```python
from build123d import *

# Parameters (mm, degrees)
SKETCH_1_R      = 4.25
EXTRUDE_1_DEPTH = 2.8
FILLET_1_R      = 0.5
SKETCH_2_W      = 14
SKETCH_2_H      = 2
EXTRUDE_2_DEPTH = 1
SKETCH_3_W      = 2
SKETCH_3_H      = 14
EXTRUDE_3_DEPTH = 1
CHAMFER_1_SIZE  = 0.5
CHAMFER_2_SIZE  = 0.5
CHAMFER_3_SIZE  = 0.5
SKETCH_4_R      = 3
EXTRUDE_4_DEPTH = 2.8


with BuildPart() as part:
    # 草图1 → 凸台-拉伸1 (new body)
    with BuildSketch(Plane(origin=(0, 0, 0), x_dir=(1, 0, 0), z_dir=(0, 1, 0))):
        with Locations(Location((0, 0, 0), (0, 0, 270))):
            Circle(SKETCH_1_R)
    extrude(amount=EXTRUDE_1_DEPTH)

    # 圆角1
    fillet_1_edges = [part.edges().sort_by_distance(p)[0] for p in [
        (0, 2.8, -4.25),
    ]]
    fillet(fillet_1_edges, radius=FILLET_1_R)

    # 草图2 → 凸台-拉伸2 (add)
    with BuildSketch(Plane.XZ):
        Rectangle(SKETCH_2_W, SKETCH_2_H)
    extrude(amount=EXTRUDE_2_DEPTH)

    # 草图3 → 凸台-拉伸3 (add)
    with BuildSketch(Plane.XZ):
        Rectangle(SKETCH_3_W, SKETCH_3_H)
    extrude(amount=EXTRUDE_3_DEPTH)

    # 倒角1
    chamfer_1_edges = [part.edges().sort_by_distance(p)[0] for p in [
        (0, 0, 7),
    ]]
    chamfer(chamfer_1_edges, length=CHAMFER_1_SIZE)

    # 倒角2
    chamfer_2_edges = [part.edges().sort_by_distance(p)[0] for p in [
        (7, 0, 0),
    ]]
    chamfer(chamfer_2_edges, length=CHAMFER_2_SIZE)

    # 倒角3
    chamfer_3_edges = [part.edges().sort_by_distance(p)[0] for p in [
        (-7, 0, 0),
        (0, 0, -7),
    ]]
    chamfer(chamfer_3_edges, length=CHAMFER_3_SIZE)

    # 草图4 → 凸台-拉伸4 (add)
    with BuildSketch(Plane.XZ.offset(1)):
        with Locations(Location((0, 0, 0), (0, 0, 70.528779366))):
            Circle(SKETCH_4_R)
    extrude(amount=EXTRUDE_4_DEPTH)


solid = part.part
```
Model file for the job. Use its own axes, mm. A direction names the side the tool comes from. Round coordinates to 2 decimals unless told otherwise and drop trailing zeros. Write each loop counter-clockwise with the first axis right and the second up, starting at its lowest first coordinate (ties: lowest second). Pieces come first, ordered by that corner, then holes. Notation, with made-up numbers: (9.5, -5) - (15.5, -5) arc R11 ccw to (15.5, 9) - close; hole circle Ø4 at (-38, -0.75). An arc over 180 degrees is marked (long way). Use CSV: the item, a comma, the result in double quotes. Start each with the question number.
Item 1: Band-saw the part on B-B (x = 0). Write the cut outline in (y, z).
Item 2: Band-saw the part on A-A (z = 0). Write the cut outline in (x, y).
Item 3: Drill centre lines: L1, parallel to Y at x = 2.5, z = -2; L2, parallel to Z at x = 2.75, y = -0.5; L3, parallel to Z at x = 2, y = 1.25. Where is each one in solid material? Low to high. Write a range as [from, to].
Item 4: Pin check, flat tips, straight feed: P1, Ø0.9, axis at x = 3, z = -3, coming from the -Y side; P2, Ø3.5, axis at x = -2, z = -3.5, coming from the -Y side; P3, Ø1.5, axis at x = 0.5, y = 0.5, coming from the -Z side; P4, Ø1.6, axis at x = -0.5, z = -5, coming from the -Y side. Stop position of each tip, or through.
Item 5: Band-saw the part on D-D (z = -5.25). Write the cut outline in (x, y).
Item 6: Tool access for faces 1 (the face through (2, 0, 2)), 2 (the face through (2, -1, -2)), 3 (the face through (-2, -1, 2)): list every direction of +Z, -Z, +X, -X, +Y, -Y with a clear straight run to the whole face (end or side of a thin tool).
Item 7: Two-plate mould, pull along Y, no slides. Class faces 4 (the face through (0, -1, -5)), 5 (the face through (4, -0.5, -1)), 6 (the face through (5, 0, 0)): released by +Y, released by -Y, zero draft, split by the parting line, or undercut.
Item 8: Band-saw the part on C-C (y = -2). Write the cut outline in (x, z).
Checked values:
1,outline,"(-3.8, -3) - (-1, -3) - (-1, -7) - (-0.5, -7) - (0, -6.5) - (0, -4.25) - (2.3, -4.25) arc R0.5 ccw to (2.8, -3.75) - (2.8, 3.75) arc R0.5 ccw to (2.3, 4.25) - (0, 4.25) - (0, 6.5) - (-0.5, 7) - (-1, 7) - (-1, 3) - (-3.8, 3) - close"
2,outline,"(-7, -1) - (-3, -1) - (-3, -3.8) - (3, -3.8) - (3, -1) - (7, -1) - (7, -0.5) - (6.5, 0) - (4.25, 0) - (4.25, 2.3) arc R0.5 ccw to (3.75, 2.8) - (-3.75, 2.8) arc R0.5 ccw to (-4.25, 2.3) - (-4.25, 0) - (-6.5, 0) - (-7, -0.5) - close"
3,L1,"y = [0, 2.8]"
3,L2,"z = [-1, 1]"
3,L3,"z = [-3.75, 3.75]"
4,P1,"stops at y = 0"
4,P2,"stops at y = -3.8"
4,P3,"stops at z = -6.75"
4,P4,"stops at y = -1"
5,outline,"(-1, -1) - (1, -1) - (1, 0) - (-1, 0) - close"
6,face 1,"+Z, +X"
6,face 2,"-Z, +X"
6,face 3,"+Z, -X"
7,face 4,"released by -Y"
7,face 5,"undercut"
7,face 6,"released by +Y"
8,outline,"circle Ø6 at (0, 0)"
